Work out the finished part from the listing and answer in its coordinate system (mm). Face numbers are marked on the shaded views. A direction names the side the tool comes from. Coordinates: 2 decimals unless noted, no trailing zeros. Loops run counter-clockwise (first coordinate to the right, second up) from the corner with the lowest first, then second, coordinate; pieces in that order, holes last. Notation, with made-up numbers: M 45.5,37.5 L 55.5,37.5 A25 ccw 55.5,52.5 Z; hole C 75,-3.75 d11. An arc over 180 degrees is marked long. Write each question's results on one line, items separated by ' | '.
Autodesk Inventor part; units mm, degrees
ref_plane "YZ Plane" through (0, 0, 0) normal (1, 0, 0) x (0, 1, 0)
ref_plane "XZ Plane" through (0, 0, 0) normal (0, 1, 0) x (-1, 0, 0)
ref_plane "XY Plane" through (0, 0, 0) normal (0, 0, 1) x (1, 0, 0)
sketch "Sketch1" plane through (0, 0, 0) normal (0, 0, 1) x (1, 0, 0)
  point P0 (0, 0)
sketch "Sketch2" plane through (0, 0, 0) normal (0, 0, 1) x (1, 0, 0)
  line L0 (12.1777, -1.5396) -> (4.6777, -1.5396) construction
  line L1 (4.6777, -1.5396) -> (4.6777, -5.5396) construction
  line L2 (4.6777, -5.5396) -> (12.1777, -5.5396) construction
  line L3 (12.1777, -5.5396) -> (12.1777, -1.5396) construction
  line L4 (8.4277, -4.7896) -> (12.4277, -4.7896)
  line L5 (12.4277, -4.7896) -> (12.4277, -2.2896)
  line L6 (12.4277, -2.2896) -> (8.4277, -2.2896)
  line L7 (8.4277, -2.2896) -> (8.4277, -4.7896)
  line L8 (8.4277, -2.2896) -> (8.4277, -8.9787)
  line L9 (8.4277, -8.9787) -> (10.4777, -8.9787)
  line L10 (10.4777, -8.9787) -> (10.4777, -4.7896)
  line L11 (9.1419, -2.2896) -> (9.1419, -1.5396) construction
  line L12 (9.1419, -4.7896) -> (9.1419, -5.5396) construction
  point P0 (0, 0)
  dimension "d0" = 7.5
  dimension "d1" = 4
  dimension "d2" = 8
  dimension "d3" = 2.5
  dimension "d4" = 4.1
  dimension "d6" = 0.75
revolve "Revolution1" add sketch "Sketch2" angle 360 about axis through (8.4277, -2.2896, 0) along (0, -1, 0)
sketch "Sketch3" plane through (8.4277, -8.9787, 0) normal (0, -1, 0) x (1, 0, 0)
  line L0 (6, 3.75) -> (-6, 3.75)
  line L1 (-6, 3.75) -> (-6, -3.75)
  line L2 (-6, -3.75) -> (6, -3.75)
  line L3 (6, -3.75) -> (6, 3.75)
  line L4 (6, 3.75) -> (-6, -3.75) construction
  line L5 (-6, 3.75) -> (6, -3.75) construction
  circle A0 centre (0, 0) radius 2.05
  point P0 (-8.4277, 0)
  point P1 (0, 0)
  dimension "d7" = 12
  dimension "d8" = 7.5
extrude "Extrusion1" add sketch "Sketch3" along normal blind 12 contours L3 L2 L1 L0 | A0
sketch "Sketch4" plane through (14.4277, -8.9787, -3.75) normal (0, 0, -1) x (-1, 0, 0)
  line L0 (12, 0) -> (0, 0)
  line L1 (0, 0) -> (0, -12)
  line L2 (12, -12) -> (0, -12)
  line L3 (12, 0) -> (12, -12)
  circle A0 centre (6, -6) radius 6
  point P0 (14.4277, 8.9787)
  point P1 (0, -6)
  point P2 (6, 0)
  point P3 (12, -6)
  point P4 (6, -12)
extrude "Extrusion2" cut sketch "Sketch4" against normal blind 12 contours L3 A0 L0 | A0 L1 L0 | L3 L2 A0 | A0 L2 L1
sketch "Sketch6" plane through (0, 0, 0) normal (0, 0, 1) x (1, 0, 0)
  circle A0 centre (8.4277, -14.9787) radius 6
  circle A1 centre (8.4277, -14.9787) radius 3
  point P0 (0, 0)
  dimension "d13" = 6
extrude "Extrusion3" cut sketch "Sketch6" along normal mid plane 3 contours A1
sketch "Sketch7" plane through (8.4277, -14.9787, 1.5) normal (0, 0, -1) x (-1, 0, 0)
  circle A0 centre (0, 0) radius 3
  circle A1 centre (0, 0) radius 4.5
  point P0 (8.4277, 14.9787)
  dimension "d16" = 9
extrude "Extrusion4" cut sketch "Sketch7" against normal blind 8.25 contours A0 | A1
sketch "Sketch8" plane through (8.4277, -14.9787, -1.5) normal (0, 0, 1) x (1, 0, 0)
  circle A0 centre (0, 0) radius 4.5
  point P0 (-8.4277, 14.9787)
extrude "Extrusion5" cut sketch "Sketch8" against normal blind 8.25
sketch "Sketch9" plane through (8.4277, -2.2896, 0) normal (0, 1, 0) x (1, 0, 0)
  circle A0 centre (0, 0) radius 4
  line L0 (3.75, -3.75) -> (-3.75, -3.75)
  line L1 (-3.75, -3.75) -> (-3.75, 3.75)
  line L2 (-3.75, 3.75) -> (3.75, 3.75)
  line L3 (3.75, 3.75) -> (3.75, -3.75)
  line L4 (3.75, -3.75) -> (-3.75, 3.75) construction
  line L5 (-3.75, -3.75) -> (3.75, 3.75) construction
  point P0 (-3.75, -1.3919)
  point P1 (-3.75, 1.3919)
  point P2 (1.3919, -3.75)
  point P3 (-1.3919, -3.75)
  point P4 (3.75, 1.3919)
  point P5 (3.75, -1.3919)
  point P6 (-1.3919, 3.75)
  point P7 (1.3919, 3.75)
  dimension "d23" = 7.5
extrude "Extrusion6" cut sketch "Sketch9" against normal up to surface (2.5 mm away) contours A0 L3 | L2 A0 | A0 L0 | L1 A0
sketch "Sketch10" plane through (8.4277, -8.9787, 0) normal (0, -1, 0) x (1, 0, 0)
  line L0 (-1.3919, 3.75) -> (1.3919, 3.75)
  arc A0 (3.75, 1.3919) -> (1.3919, 3.75) centre (0, 0) ccw
  line L1 (3.75, 1.3919) -> (3.75, -1.3919)
  arc A1 (1.3919, -3.75) -> (3.75, -1.3919) centre (0, 0) ccw
  line L2 (1.3919, -3.75) -> (-1.3919, -3.75)
  arc A2 (-3.75, -1.3919) -> (-1.3919, -3.75) centre (0, 0) ccw
  line L3 (-3.75, -1.3919) -> (-3.75, 1.3919)
  arc A3 (-1.3919, 3.75) -> (-3.75, 1.3919) centre (0, 0) ccw
  circle A4 centre (0, 0) radius 2.05
  point P0 (-8.4277, 0)
extrude "Extrusion7" add sketch "Sketch10" along normal up to surface contours A4
properties part number "Sholder"
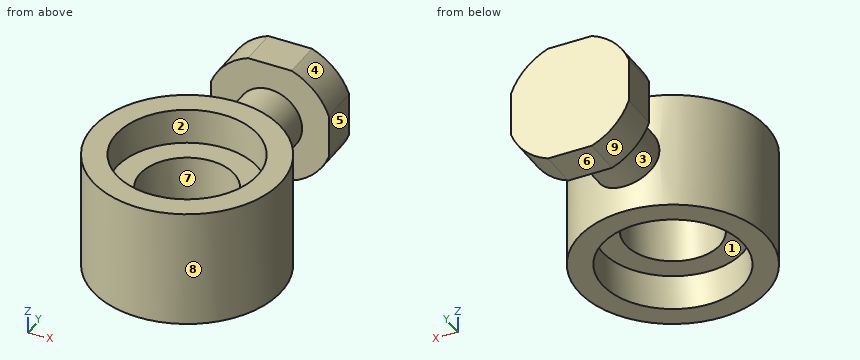
1) For a pull along X with two mould halves and no side action, classify the marked faces 6, 7, 8 and 9 as released by +X, released by -X, zero draft, split by the parting line, or undercut.
Check result:
face 6: zero draft | face 7: undercut | face 8: split by the parting line | face 9: released by -X
2) Which of the six approach directions +Z, -Z, +X, -X, +Y, -Y give full straight-line access (tool end or side, diameter ignored) to the marked faces 1, 2, 3, 4 and 5?
Check result:
face 1: -Z | face 2: +Z | face 3: none | face 4: +Z, +X, +Y | face 5: +Z, -Z, +X, +Y
3) Straight lines are drawn through the part: probe 1 along Y at (x, z) = (6, -1); probe 2 along Y at (x, z) = (8.5, 0.5); probe 3 along Y at (x, z) = (5, -3). For each, find the intervals that lie inside material, in ascending order. Write a range as [from, to].
Check result:
probe 1: [-20.47, -16.74], [-13.22, -9.49], [-4.79, -2.29] | probe 2: [-20.98, -17.98], [-11.98, -2.29] | probe 3: [-19.9, -17.89], [-12.06, -10.05]
4) Find section A-A, the plane z = 3.25. Give the vertices of the cut face in (x, y).
Check result:
outline: C 8.43,-14.98 d12; M 6.1,-4.79 L 10.76,-4.79 L 10.76,-2.29 L 6.1,-2.29 Z; hole C 8.43,-14.98 d9
5) Find section B-B, the plane y = -14.5. Give the vertices of the cut face in (x, z), and give its area (3 significant figures).
Check result:
outline: M 2.45,-3.75 L 3.95,-3.75 L 3.95,-1.5 L 5.47,-1.5 L 5.47,1.5 L 3.95,1.5 L 3.95,3.75 L 2.45,3.75 Z; M 11.39,-1.5 L 12.9,-1.5 L 12.9,-3.75 L 14.41,-3.75 L 14.41,3.75 L 12.9,3.75 L 12.9,1.5 L 11.39,1.5 Z | area: 31.7 mm^2
6) Find section D-D, the plane y = -16.75. Give the vertices of the cut face in (x, z).
Check result:
outline: M 2.7,-3.75 L 4.29,-3.75 L 4.29,-1.5 L 6.01,-1.5 L 6.01,1.5 L 4.29,1.5 L 4.29,3.75 L 2.7,3.75 Z; M 10.85,-1.5 L 12.56,-1.5 L 12.56,-3.75 L 14.16,-3.75 L 14.16,3.75 L 12.56,3.75 L 12.56,1.5 L 10.85,1.5 Z
7) Given pin 1 Ø4 at (x, y) = (6.5, -8.5) entering from +Z; pin 2 Ø2 at (x, y) = (9, -12.5) entering from +Z; pin 3 Ø2 at (y, z) = (-3.5, 0) entering from +X; pin 4 Ø3 at (y, z) = (-18, 1.5) entering from +X, each flat-ended and moving along its own axis, determine where each tip first touches the part or whether it passes through.
Check result:
pin 1: z = 3.75 | pin 2: z = 1.5 | pin 3: x = 12.18 | pin 4: x = 14.23
